from build123d import *

# Parameters (mm, degrees)
SKETCH1_W                      = 158
SKETCH1_H                      = 199.5
BOSS_EXTRUDE1_DEPTH            = 6.35
BOSS_EXTRUDE2_DEPTH            = 12.7
CBORE_FOR_M4_SHCS1_D           = 4.5
CBORE_FOR_M4_SHCS1_DEPTH       = 6.35
CBORE_FOR_M4_SHCS1_CBORE_D     = 8
CBORE_FOR_M4_SHCS1_CBORE_DEPTH = 4
FILLET4_R                      = 5
SKETCH17_W                     = 20
SKETCH17_H                     = 159
BOSS_EXTRUDE3_DEPTH            = 6.35
SKETCH18_R                     = 3
ENCLOSURE_DEPTH                = 7.35
SKETCH19_R                     = 2.5
CUT_EXTRUDE4_DEPTH             = 7.35
SKETCH20_R                     = 3.05
CUT_EXTRUDE5_DEPTH             = 3.1


with BuildPart() as part:
    # Sketch1 → Boss-Extrude1 (new body)
    with BuildSketch(Plane(origin=(0, 0, 0), x_dir=(1, 0, 0), z_dir=(0, 1, 0))):
        with Locations((79, -99.75)):
            Rectangle(SKETCH1_W, SKETCH1_H)
    extrude(amount=BOSS_EXTRUDE1_DEPTH)

    # Sketch3 → Boss-Extrude2 (add)
    with BuildSketch(Plane(origin=(0, 6.35, 0), x_dir=(1, 0, 0), z_dir=(0, 1, 0))):
        Polygon((158, -199.5), (158, 0), (153, 0), (153, -194.5), (0, -194.5), (0, -199.5), align=None)
    extrude(amount=BOSS_EXTRUDE2_DEPTH)

    # CBORE for M4 SHCS1
    with Locations(Plane(origin=(0, 6.35, 0), x_dir=(1, 0, 0), z_dir=(0, 1, 0))):
        with Locations((138, -55), (20, -179.5), (60, -179.5), (138, -130), (138, -105), (138, -30)):
            CounterBoreHole(CBORE_FOR_M4_SHCS1_D / 2, CBORE_FOR_M4_SHCS1_CBORE_D / 2, CBORE_FOR_M4_SHCS1_CBORE_DEPTH, depth=CBORE_FOR_M4_SHCS1_DEPTH)

    # Fillet4
    fillet4_edges = [part.edges().sort_by_distance(p)[0] for p in [
        (158, 9.525, 199.5),
    ]]
    fillet(fillet4_edges, radius=FILLET4_R)

    # Sketch17 → Boss-Extrude3 (add)
    with BuildSketch(Plane(origin=(0, 6.35, 0), x_dir=(1, 0, 0), z_dir=(0, 1, 0))):
        with Locations((-10, -79.5)):
            Rectangle(SKETCH17_W, SKETCH17_H)
    extrude(amount=-BOSS_EXTRUDE3_DEPTH)

    # Sketch18 → Enclosure (cut, through all)
    with BuildSketch(Plane(origin=(0, 6.35, 0), x_dir=(1, 0, 0), z_dir=(0, 1, 0))):
        with Locations((13, -154.5)):
            Circle(SKETCH18_R)
        with Locations((13, -78.3)):
            Circle(SKETCH18_R)
        with Locations((140, -78.3)):
            Circle(SKETCH18_R)
        with Locations((140, -154.5)):
            Circle(SKETCH18_R)
    extrude(amount=-ENCLOSURE_DEPTH, mode=Mode.SUBTRACT)

    # Sketch19 → Cut-Extrude4 (cut, through all)
    with BuildSketch(Plane(origin=(0, 6.35, 0), x_dir=(1, 0, 0), z_dir=(0, 1, 0))):
        with Locations((-11.75, -23)):
            Circle(SKETCH19_R)
        with Locations((127.75, -23)):
            Circle(SKETCH19_R)
    extrude(amount=-CUT_EXTRUDE4_DEPTH, mode=Mode.SUBTRACT)

    # Sketch20 → Cut-Extrude5 (cut)
    with BuildSketch(Plane(origin=(0, 6.35, 0), x_dir=(1, 0, 0), z_dir=(0, 1, 0))):
        with Locations((133, -4.25)):
            Circle(SKETCH20_R)
        with Locations((65.5, -4.25)):
            Circle(SKETCH20_R)
        with Locations((-2, -4.25)):
            Circle(SKETCH20_R)
    extrude(amount=-CUT_EXTRUDE5_DEPTH, mode=Mode.SUBTRACT)


solid = part.part
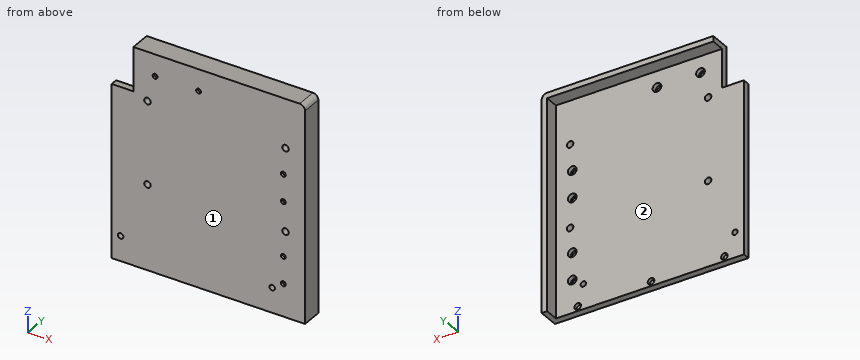
Work out the finished part from the listing and answer in its coordinate system (mm). Face numbers are marked on the shaded views. A direction names the side the tool comes from. Give positions to 0.01 mm unless a question says otherwise; leave off trailing zeros. Write each loop counter-clockwise with the first axis right and the second up, starting at its lowest first coordinate (ties: lowest second). Pieces come first, ordered by that corner, then holes. Notation, with made-up numbers: (67.5, 83.5) - (79.5, 83.5) arc R20 cw to (79.5, 107.5) - close; hole circle Ø10 at (5, -4). An arc over 180 degrees is marked (long way). One line per item, written item: value. Start each with the question number.
1. Consider probe 1 along X at (y, z) = (4.3, 4.25); probe 2 along X at (y, z) = (3.75, 78.3); probe 3 along X at (y, z) = (2.5, 23). Determine where each line is inside the solid, lowest interval first.
2. Given pin 1 (7 mm diameter, centred on x = 60, z = 179.5, fed in from +Y); pin 2 (1.5 mm diameter, centred on x = 115.5, z = 143.5, fed in from +Y), each flat-ended and moving along its own axis, determine where each tip first touches the part or whether it passes through.
3. Find section A-A (x = -11.75). Write down the section's boundary in (y, z).
4. Find section C-C (z = 55). Write down the section's boundary in (x, y), then the cut area to 3 significant figures.
5. Find section D-D (x = 127.75). Write down the section's boundary in (y, z), then the cut area to 3 significant figures.
6. For the marked faces 1 and 2, determine the directions among +Z, -Z, +X, -X, +Y, -Y from which every point of the face is accessible in a straight line to the end or side of a thin tool.
7. Find section B-B (z = 78.3). Write down the section's boundary in (x, y).
Geometry results:
1. probe 1: -20 to -5.05, 1.05 to 62.45, 68.55 to 129.95, 136.05 to 158
1. probe 2: -20 to 10, 16 to 137, 143 to 158
1. probe 3: -20 to -14.25, -9.25 to 125.25, 130.25 to 158
2. pin 1: y = 2.35
2. pin 2: y = 6.35
3. outline: (0, 0) - (6.35, 0) - (6.35, 20.5) - (0, 20.5) - close; (0, 25.5) - (6.35, 25.5) - (6.35, 159) - (0, 159) - close
4. outline: (-20, 0) - (135.75, 0) - (135.75, 2.35) - (134, 2.35) - (134, 6.35) - (-20, 6.35) - close; (140.25, 0) - (158, 0) - (158, 19.05) - (153, 19.05) - (153, 6.35) - (142, 6.35) - (142, 2.35) - (140.25, 2.35) - close
4. area: 1,150 mm2
5. outline: (0, 0) - (6.35, 0) - (6.35, 20.5) - (0, 20.5) - close; (0, 25.5) - (6.35, 25.5) - (6.35, 194.5) - (19.05, 194.5) - (19.05, 199.5) - (0, 199.5) - close
5. area: 1,300 mm2
6. face 1: +Z, -Z, +X, -X, -Y
6. face 2: -Z, -X, +Y
7. outline: (-20, 0) - (10, 0) - (10, 6.35) - (-20, 6.35) - close; (16, 0) - (137, 0) - (137, 6.35) - (16, 6.35) - close; (143, 0) - (158, 0) - (158, 19.05) - (153, 19.05) - (153, 6.35) - (143, 6.35) - close
